Source: CAD feature listing. Evaluate the final solid. Frame: model axes, mm. Face numbers are marked on the shaded views. A direction names the side the tool comes from. Give positions to 0.01 mm unless a question says otherwise; leave off trailing zeros. Write each loop counter-clockwise with the first axis right and the second up, starting at its lowest first coordinate (ties: lowest second). Pieces come first, ordered by that corner, then holes. Notation, with made-up numbers: (81.25, 37.25) - (102.25, 37.25) arc R29 ccw to (102.25, 67.25) - close; hole circle Ø6 at (48, -15). An arc over 180 degrees is marked (long way). One line per question, with ' | ' between items. Start each with the question number.
(1) Access query for the marked faces 4, 5 and 6. Directions: +Z, -Z, +X, -X, +Y, -Y. A direction counts if a zero-diameter tool reaches every point of the face in a straight line with its end or side. Return the directions, or none.
(2) Section B-B, the plane x = 25.5. Return loops of the section in (y, z).
(3) Draft query along Y for the marked faces 1, 2 and 3. Return one class per face: +Y half, -Y half, draft (parallel to the pull), parting line (faces both ways), or undercut.
(4) Pin query (flat end, axial travel): pin 1 (2.5 mm diameter, centred on y = -1, z = 0.5, fed in from +X); pin 2 (2 mm diameter, centred on x = 13.5, y = -2.5, fed in from +Z); pin 3 (3 mm diameter, centred on y = 0, z = 0, fed in from -X). Return the tip coordinate at first contact, or that it passes through.
(5) Section D-D, the plane x = 11.5. Return loops of the section in (y, z), plus the area to 3 significant figures.
(6) Ray query, line 1 (Y direction, x = 35.5, z = 0); line 2 (X direction, y = 5, z = 1.75); line 3 (Y direction, x = 35, z = -1.75). Return the intervals inside material, ascending. Write a range as [from, to].
(7) Section A-A, the plane y = 0. Return loops of the section in (x, z).
```python
from build123d import *

# Parameters (mm, degrees)
SKETCH1_R           = 4
BOSS_EXTRUDE1_DEPTH = 40
SKETCH2_R           = 2
CUT_EXTRUDE1_DEPTH  = 6
BOSS_EXTRUDE2_START = -7
SKETCH3_R           = 6
SKETCH3_R_2         = 2
BOSS_EXTRUDE2_DEPTH = 9
SKETCH4_R           = 2.4
CUT_EXTRUDE2_DEPTH  = 16


with BuildPart() as part:
    # Sketch1 → Boss-Extrude1 (new body)
    with BuildSketch(Plane(origin=(0, 0, 0), x_dir=(0, 0, -1), z_dir=(1, 0, 0))):
        Circle(SKETCH1_R)
    extrude(amount=BOSS_EXTRUDE1_DEPTH)

    # Sketch2 → Cut-Extrude1 (cut)
    with BuildSketch(Plane.ZY):
        Circle(SKETCH2_R)
    extrude(amount=-CUT_EXTRUDE1_DEPTH, mode=Mode.SUBTRACT)

    # Sketch3 → Boss-Extrude2 (add)
    with BuildSketch(Plane.ZY.offset(BOSS_EXTRUDE2_START)):
        Circle(SKETCH3_R)
        Circle(SKETCH3_R_2, mode=Mode.SUBTRACT)
    extrude(amount=-BOSS_EXTRUDE2_DEPTH)

    # Sketch4 → Cut-Extrude2 (cut)
    with BuildSketch(Plane(origin=(40, 0, 0), x_dir=(0, 0, -1), z_dir=(1, 0, 0))):
        Circle(SKETCH4_R)
    extrude(amount=-CUT_EXTRUDE2_DEPTH, mode=Mode.SUBTRACT)


solid = part.part
```
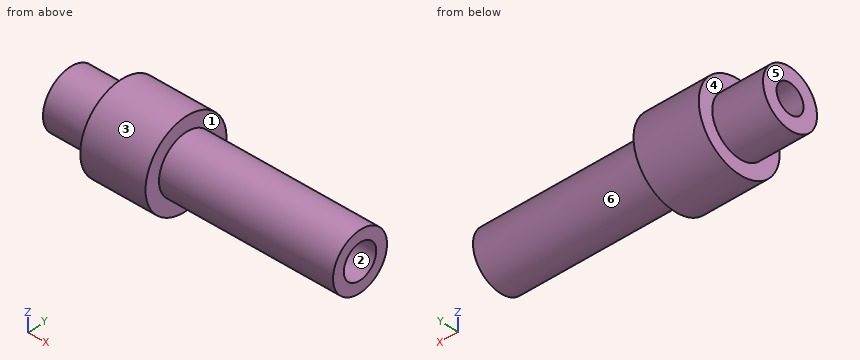
Check sheet entries:
1) face 4: -X | face 5: +Z, -Z, -X, +Y, -Y | face 6: +X
2) outline: circle Ø8 at (0, 0); hole circle Ø4.8 at (0, 0)
3) face 1: draft | face 2: undercut | face 3: parting line
4) pin 1: x = 24 | pin 2: z = 5.81 | pin 3: x = 6
5) outline: circle Ø12 at (0, 0) | area: 113 mm²
6) line 1: [-4, -2.4], [2.4, 4] | line 2: [7, 16] | line 3: [-3.6, -1.64], [1.64, 3.6]
7) outline: (0, -4) - (7, -4) - (7, -6) - (16, -6) - (16, -4) - (40, -4) - (40, -2.4) - (24, -2.4) - (24, 2.4) - (40, 2.4) - (40, 4) - (16, 4) - (16, 6) - (7, 6) - (7, 4) - (0, 4) - (0, 2) - (6, 2) - (6, -2) - (0, -2) - close
